Work out the finished part from the listing and answer in its coordinate system (mm). Round coordinates to 2 decimals unless told otherwise and drop trailing zeros. Order: outer loops, then holes, each group sorted by start corner. A loop starts at its lowest first (then second) coordinate and runs counter-clockwise, first axis right, second up. Notation, with made-up numbers: (80, 89.5) -> (100, 89.5) arc R21 cw to (100, 97.5) -> close; hole circle Ø2 at (-37.75, 1.5). An arc over 180 degrees is marked (long way). Use one line per item in the form item = value.
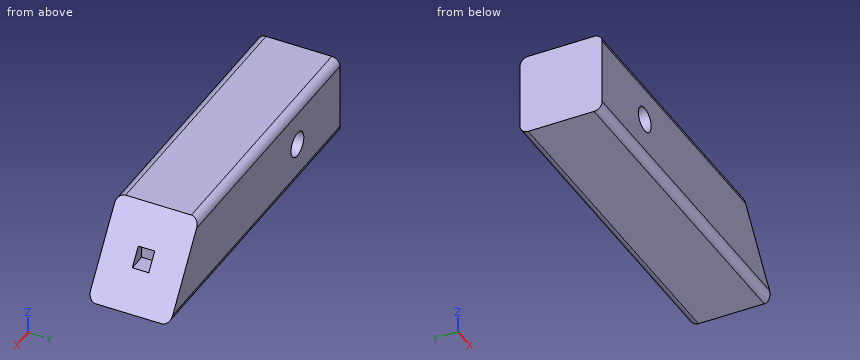
```python
from build123d import *

# Parameters (mm, degrees)
F0_W     = 127
F0_H     = 31.75
F1_DEPTH = 15.875
F2_R     = 4.7625
F3_DEPTH = 31.751
F5_DEPTH = 31.751
F7_W     = 6.35
F7_H     = 6.35
F8_DEPTH = 15.875
F9_R     = 3.175


with BuildPart() as f1:
    # F0 (on Front) → F1 (new body, symmetric)
    with BuildSketch(Plane.XZ):
        Rectangle(F0_W, F0_H)
    extrude(amount=F1_DEPTH, both=True)

    # F2 (on face) → F3 (cut, through all)
    with BuildSketch(Plane.XZ.offset(15.875)):
        with Locations((-31.75, 0)):
            Circle(F2_R)
    extrude(amount=-F3_DEPTH, mode=Mode.SUBTRACT)

    # F4 (on face) → F5 (cut, through all)
    with BuildSketch(Plane.XZ.offset(15.875)):
        Polygon((41.2684106618, 15.875), (63.5, -15.875), (63.5, 15.875), align=None)
    extrude(amount=-F5_DEPTH, mode=Mode.SUBTRACT)

    # F7 (on offset) → F8 (cut)
    with BuildSketch(Plane.YZ.offset(63.5)):
        Rectangle(F7_W, F7_H)
    extrude(amount=-F8_DEPTH, mode=Mode.SUBTRACT)

    # F9
    f9_edges = [f1.edges().sort_by_distance(p)[0] for p in [
        (-11.115795, -15.875, 15.875),
        (-11.115795, 15.875, 15.875),
        (0, -15.875, -15.875),
        (0, 15.875, -15.875),
    ]]
    fillet(f9_edges, radius=F9_R)


solid = f1.part
```
Item 1: Flat-ended cylindrical pins translate along their axes: P1, Ø3, axis at x = 52.5, y = 1.5, coming from the +Z side (3 decimals); P2, Ø7, axis at y = 0, z = -0.5, coming from the +X side; P3, Ø1.5, axis at y = -6.5, z = 7, coming from the +X side. Find the tip coordinate at first contact, or state that the pin passes through.
Findings:
P1 = -3.175
P2 = 55.19
P3 = 48.01
Item 2: The part is cut by section C-C, the plane z = 0. Give the vertices of the cut face in (x, y) (1 decimal), and give its area (3 significant figures).
Findings:
outline = (-63.5, -15.9) -> (-36.5, -15.9) -> (-36.5, 15.9) -> (-63.5, 15.9) -> close; (-27, -15.9) -> (52.4, -15.9) -> (52.4, -3.2) -> (47.6, -3.2) -> (47.6, 3.2) -> (52.4, 3.2) -> (52.4, 15.9) -> (-27, 15.9) -> close
area = 3,350 mm^2
Item 3: Consider line 1 along Z through (x, y) = (-31.75, 4.5) (1 decimal); line 2 along X through (y, z) = (-5, 3.5); line 3 along Z through (x, y) = (-31, -4) (3 decimals). Determine where each line is inside the solid, lowest interval first.
Findings:
line_1 = -15.9 to -4.8, 4.8 to 15.9
line_2 = -63.5 to -34.98, -28.52 to 49.93
line_3 = -15.875 to -4.703, 4.703 to 15.875
